Work out the finished part from the listing and answer in its coordinate system (mm). Face numbers are marked on the shaded views. Coordinates: 2 decimals unless noted, no trailing zeros. Loops run counter-clockwise (first coordinate to the right, second up) from the corner with the lowest first, then second, coordinate; pieces in that order, holes last. Notation, with made-up numbers: (29.5, 74.25) - (38.5, 74.25) arc R16 cw to (38.5, 100.25) - close; hole circle Ø1 at (34.25, 49.5). An arc over 180 degrees is marked (long way). Write each question's results on one line, items separated by ' | '. Start each with the question number.
Item 1: Consider probe 1 along X at (y, z) = (188.5, 21.25); probe 2 along X at (y, z) = (147.5, 4.5); probe 3 along Y at (x, z) = (55.5, 20.5). Determine where each line is inside the solid, lowest interval first. Write a range as [from, to].
Item 2: Section A-A, the plane y = 182 is taken. Write down the section's boundary in (x, z), plus the area to 3 significant figures.
Item 3: Section C-C, the plane x = -83.5 is taken. Write down the section's boundary in (y, z), plus the area to 3 significant figures.
Item 4: Section D-D, the plane z = 15 is taken. Write down the section's boundary in (x, y) (3 decimals).
Item 5: Each of these flat-tipped pins is pushed along its axis until it touches: pin 1 Ø4.5 at (y, z) = (174.5, 16) entering from -X; pin 2 Ø4.5 at (x, z) = (-77, 9.5) entering from -Y. Where does it stop, or does it pass through?
Item 6: Section B-B, the plane y = 108 is taken. Write down the section's boundary in (x, z).
Item 7: For a pull along X with two mould halves and no side action, classify the marked faces 1 and 2 as +X half, -X half, draft (parallel to the pull), parting line (faces both ways), or undercut.
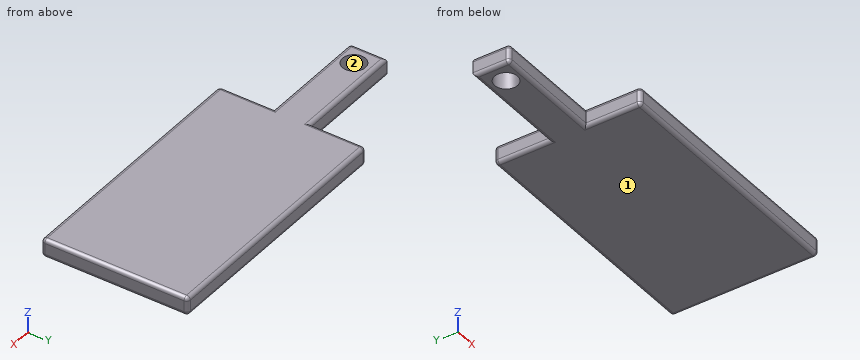
from build123d import *

# Parameters (mm, degrees)
F0_W     = 152.4
F0_H     = 50.8
F1_DEPTH = 25.4
F2_R     = 15.875
F4_DEPTH = 25.401
F5_R     = 5.08


with BuildPart() as f1:
    # F0 (on Top) → F1 (new body)
    with BuildSketch(Plane.XY):
        Polygon((0, 76.2), (0, 0), (355.6, 0), (355.6, 203.2), (0, 203.2), (0, 127), align=None)
        with Locations((-76.2, 101.6)):
            Rectangle(F0_W, F0_H)
    extrude(amount=F1_DEPTH)

    # F2 (on face) → F4 (cut, through all)
    with BuildSketch(Plane.XY.offset(25.4)):
        with Locations((-123.832056, 100.965)):
            Circle(F2_R)
    extrude(amount=-F4_DEPTH, mode=Mode.SUBTRACT)

    # F5
    f5_edges = [f1.edges().sort_by_distance(p)[0] for p in [
        (-152.4, 76.2, 12.7),
        (-76.2, 127, 25.4),
        (-152.4, 101.6, 25.4),
        (-76.2, 76.2, 25.4),
        (-76.2, 76.2, 0),
        (0, 38.1, 25.4),
        (0, 165.1, 25.4),
        (177.8, 203.2, 25.4),
        (177.8, 0, 25.4),
        (177.8, 0, 0),
        (0, 0, 12.7),
        (355.6, 101.6, 25.4),
        (355.6, 0, 12.7),
        (355.6, 101.6, 0),
        (355.6, 203.2, 12.7),
        (177.8, 203.2, 0),
        (0, 38.1, 0),
        (0, 165.1, 0),
        (0, 203.2, 12.7),
        (-152.4, 101.6, 0),
        (-76.2, 127, 0),
    ]]
    fillet(f5_edges, radius=F5_R)


solid = f1.part
Answer key:
1) probe 1: x = [0.09, 355.51] | probe 2: x = [0.03, 355.57] | probe 3: y = [0, 203.2]
2) outline: (0, 5.08) arc R5.08 ccw to (5.08, 0) - (350.52, 0) arc R5.08 ccw to (355.6, 5.08) - (355.6, 20.32) arc R5.08 ccw to (350.52, 25.4) - (5.08, 25.4) arc R5.08 ccw to (0, 20.32) - close | area: 9,010 mm^2
3) outline: (76.2, 5.08) arc R5.08 ccw to (81.28, 0) - (121.92, 0) arc R5.08 ccw to (127, 5.08) - (127, 20.32) arc R5.08 ccw to (121.92, 25.4) - (81.28, 25.4) arc R5.08 ccw to (76.2, 20.32) - close | area: 1,270 mm^2
4) outline: (-152.4, 81.28) arc R5.08 ccw to (-147.32, 76.2) - (0, 76.2) - (0, 5.08) arc R5.08 ccw to (5.08, 0) - (350.52, 0) arc R5.08 ccw to (355.6, 5.08) - (355.6, 198.12) arc R5.08 ccw to (350.52, 203.2) - (5.08, 203.2) arc R5.08 ccw to (0, 198.12) - (0, 127) - (-152.4, 127) - close; hole circle Ø31.75 at (-123.832, 100.965)
5) pin 1: stops at x = 0 | pin 2: stops at y = 76.2
6) outline: (-152.4, 5.08) arc R5.08 ccw to (-147.32, 0) - (-138.06, 0) - (-138.06, 25.4) - (-147.32, 25.4) arc R5.08 ccw to (-152.4, 20.32) - close; (-109.6, 0) - (350.52, 0) arc R5.08 ccw to (355.6, 5.08) - (355.6, 20.32) arc R5.08 ccw to (350.52, 25.4) - (-109.6, 25.4) - close
7) face 1: draft | face 2: undercut
